Check sheet for the modelled part. Datum: model origin and axes. Units: mm. A direction names the side the tool comes from. Round coordinates to 2 decimals unless told otherwise and drop trailing zeros. Write each loop counter-clockwise with the first axis right and the second up, starting at its lowest first coordinate (ties: lowest second). Pieces come first, ordered by that corner, then holes. Notation, with made-up numbers: (13.5, 69.5) -> (64.5, 69.5) arc R35 cw to (64.5, 104.5) -> close; hole circle Ø10 at (-16.5, 43.25). An arc over 180 degrees is marked (long way). One line per item, written item: value.
Autodesk Inventor part; units mm, degrees
ref_plane "YZ Plane" through (0, 0, 0) normal (1, 0, 0) x (0, 1, 0)
ref_plane "XZ Plane" through (0, 0, 0) normal (0, 1, 0) x (-1, 0, 0)
ref_plane "XY Plane" through (0, 0, 0) normal (0, 0, 1) x (1, 0, 0)
sketch "Skizze1" plane through (0, 0, 0) normal (0, 1, 0) x (-1, 0, 0)
  line L0 (35, 52.5) -> (-35, 52.5)
  line L1 (-35, 52.5) -> (-35, -52.5)
  line L2 (-35, -52.5) -> (35, -52.5)
  line L3 (35, -52.5) -> (35, 52.5)
  point P0 (0, 0)
  point P1 (35, 0)
  point P2 (0, 52.5)
  dimension "d0" = 70
  dimension "d1" = 105
extrude "Extrusion1" add sketch "Skizze1" along normal blind 2
sketch "Skizze3" plane through (0, 2, 0) normal (0, 1, 0) x (1, 0, 0)
  line L0 (31, 48.5) -> (-31, 48.5) construction
  line L1 (-31, 48.5) -> (-31, -48.5) construction
  line L2 (-31, -48.5) -> (31, -48.5) construction
  line L3 (31, -48.5) -> (31, 48.5) construction
  line L4 (35, -52.5) -> (35, 52.5) construction
  line L5 (35, 52.5) -> (-35, 52.5) construction
  line L6 (-35, 52.5) -> (-35, -52.5) construction
  line L7 (-35, -52.5) -> (35, -52.5) construction
  point P0 (0, 0)
  point P1 (31, 0)
  point P2 (0, 48.5)
  dimension "d27" = 105
  dimension "d28" = 70
  dimension "d29" = 62
  dimension "d30" = 97
hole "Bohrung1" at (31, 2, 48.5) at (-31, 2, 48.5) at (-31, 2, -48.5) at (31, 2, -48.5) direction (0, -1, 0) diameter 3 end through all
sketch "Skizze5" plane through (0, 2, 0) normal (0, 1, 0) x (1, 0, 0)
  line L0 (0, 40.5) -> (-2, 40.5)
  line L1 (-2, 40.5) -> (-2, 20.5)
  line L2 (-2, 20.5) -> (0, 20.5)
  line L3 (0, 20.5) -> (0, 40.5)
  line L4 (0, 10.5) -> (-7, 10.5)
  line L5 (-7, 10.5) -> (-7, 8.5)
  line L6 (-7, 8.5) -> (0, 8.5)
  line L7 (0, 8.5) -> (0, 10.5)
  circle A0 centre (-31, 48.5) radius 1.5 construction
  circle A1 centre (31, -48.5) radius 1.5 construction
  circle A2 centre (-31, -48.5) radius 1.5 construction
  circle A3 centre (31, 48.5) radius 1.5 construction
  line L8 (35, -52.5) -> (35, 52.5) construction
  line L9 (35, 52.5) -> (-35, 52.5) construction
  line L10 (-35, 52.5) -> (-35, -52.5) construction
  line L11 (-35, -52.5) -> (35, -52.5) construction
  line L12 (-7, 20.5) -> (-5, 20.5)
  line L13 (-5, 20.5) -> (-5, 40.5)
  line L14 (-5, 40.5) -> (-7, 40.5)
  line L15 (-7, 40.5) -> (-7, 20.5)
  point P0 (0, 0)
  point P1 (-1, 20.5)
  dimension "d45" = 2
  dimension "d46" = 42
  dimension "d48" = 20
  dimension "d49" = 7
  dimension "d51" = 0
  dimension "d56" = 10
  dimension "d57" = 3
  dimension "d58" = 20
  dimension "d59" = 0
extrude "Extrusion5" [suppressed]
sketch "Skizze6" plane through (0, 2, 0) normal (0, 1, 0) x (1, 0, 0)
  line L0 (-17.5, 17.5) -> (17.5, 17.5) construction
  line L1 (17.5, 17.5) -> (17.5, -17.5) construction
  line L2 (17.5, -17.5) -> (-17.5, -17.5) construction
  line L3 (-17.5, -17.5) -> (-17.5, 17.5) construction
  circle A0 centre (-17.5, 17.5) radius 3
  circle A1 centre (-17.5, -17.5) radius 3
  circle A2 centre (17.5, -17.5) radius 3
  circle A3 centre (17.5, 17.5) radius 3
  point P0 (0, 0)
  point P1 (-17.5, 0)
  point P2 (0, 17.5)
  dimension "d60" = 35
  dimension "d61" = 6
  dimension "d62" = 6
  dimension "d63" = 6
  dimension "d64" = 6
extrude "Extrusion6" add sketch "Skizze6" along normal blind 6
sketch "Skizze7" plane through (0, 0, 0) normal (0, -1, 0) x (1, 0, 0)
  circle A0 centre (-17.5, 17.5) radius 3 construction
  circle A1 centre (-17.5, -17.5) radius 3 construction
  arc A2 (20.5, -17.5) -> (20.5, -17.5) centre (17.5, -17.5) ccw construction
  arc A3 (20.5, 17.5) -> (20.5, 17.5) centre (17.5, 17.5) ccw construction
  point P0 (0, 0)
  point P1 (20, -17.5)
  point P2 (20, 17.5)
hole "Bohrung2" at (-17.5, 0, 17.5) at (-17.5, 0, -17.5) at (17.5, 0, -17.5) at (17.5, 0, 17.5) direction (0, 1, 0) diameter 2.5 depth 5 tip angle 118
chamfer "Fase1" distance 1 angle 45 4 edges at (-35, 1, 52.5) (35, 1, 52.5) (35, 1, -52.5) (-35, 1, -52.5)
sketch "Skizze10" plane through (0, 0, 0) normal (0, -1, 0) x (1, 0, 0)
  point P0 (0, 0)
  point P1 (-3, -41)
  point P2 (-6, -41)
  point P3 (-9, -41)
  dimension "d105" = 41
  dimension "d106" = 3
  dimension "d107" = 3
  dimension "d108" = 3
hole "Bohrung3" at (-3, 0, -41) at (-6, 0, -41) at (-9, 0, -41) direction (0, 1, 0) diameter 1.5 depth 5 tip angle 118
pattern_circular "Runde Anordnung1" count 7 over 360 about axis through (-3, 2.5, -41) along (0, -1, 0) of "Bohrung3"
equation "\"d62\" = d61"
equation "\"d63\" = d61"
equation "\"d64\" = d61"
properties part number "Case_bottom" material "PC/ABS-Kunststoff"
Item 1: Tool access check on faces 1 (the cylindrical face through (31, 1, -50)), 2 (the cylindrical face through (17.12, 2.54, 16.31)), 3 (the cylindrical face through (-19.9, 5, -19.3)). Record the directions out of +Z, -Z, +X, -X, +Y, -Y that give a thin tool (end or side, any length) a straight path to the whole face; none if there is none.
Result set:
face 1: +Y, -Y
face 2: -Y
face 3: +Y
Item 2: Sectioned sample at A-A (y = 3.5). Enter the section's corners in (x, z), then the cut area to 3 significant figures.
Result set:
outline: circle Ø6 at (-17.5, -17.5); circle Ø6 at (-17.5, 17.5); circle Ø6 at (17.5, -17.5); circle Ø6 at (17.5, 17.5); hole circle Ø2.5 at (-17.5, -17.5); hole circle Ø2.5 at (-17.5, 17.5); hole circle Ø2.5 at (17.5, -17.5); hole circle Ø2.5 at (17.5, 17.5)
area: 93.5 mm^2
Item 3: Depth check by flat-ended pin: pin 1 (4 mm diameter, centred on x = -17, y = 6, fed in from +Z); pin 2 (5 mm diameter, centred on x = 17.5, z = 40.5, fed in from -Y); pin 3 (5 mm diameter, centred on x = -8.5, z = -1.5, fed in from +Y). Enter the tip coordinate at first touch or a pass-through.
Result set:
pin 1: z = 20.5
pin 2: y = 0
pin 3: y = 2
Item 4: Release check for a two-part mould opening along Z. For faces 4 (the flat face through (-18, 8, -18)), 5 (the flat face through (0, 1, 52.5)), 6 (the cylindrical face through (15.1, 5, -19.3)) record: pulls with the +Z half, pulls with the -Z half, needs draft (parallel to the pull), parting line crosses it, or undercut.
Result set:
face 4: needs draft
face 5: pulls with the +Z half
face 6: undercut
Item 5: Sectioned sample at D-D (z = -11.5). Enter the section's corners in (x, y).
Result set:
outline: (-35, 0) -> (35, 0) -> (35, 2) -> (-35, 2) -> close
Item 6: Sectioned sample at B-B (x = 31). Enter the section's corners in (y, z), then the cut area to 3 significant figures.
Result set:
outline: (0, -52.5) -> (2, -52.5) -> (2, -50) -> (0, -50) -> close; (0, -47) -> (2, -47) -> (2, 47) -> (0, 47) -> close; (0, 50) -> (2, 50) -> (2, 52.5) -> (0, 52.5) -> close
area: 198 mm^2
Item 7: Material ranges on line 1 along Z through (x, y) = (17.5, 2.2); line 2 along X through (y, z) = (1.15, -48.5); line 3 along Y through (x, z) = (-2.5, 30.5), recorded low to high.
Result set:
line 1: -20.5 to -18.75, -16.25 to -14.5, 14.5 to 16.25, 18.75 to 20.5
line 2: -35 to -32.5, -29.5 to 29.5, 32.5 to 35
line 3: 0 to 2
Item 8: Sectioned sample at C-C (x = -28). Enter the section's corners in (y, z), then the cut area to 3 significant figures.
Result set:
outline: (0, -52.5) -> (2, -52.5) -> (2, 52.5) -> (0, 52.5) -> close
area: 210 mm^2
